Input: part model. Units: mm. Frame: model coordinates. Round coordinates to 2 decimals unless told otherwise and drop trailing zeros. Loops run counter-clockwise (first coordinate to the right, second up) from the corner with the lowest first, then second, coordinate; pieces in that order, holes last.
(1) Cut plane A-A, the plane z = -3. Output: boundary loops of the cut face in (x, y).
(2) Draft query along X for faces 1 (the face through (0.08, -17.996, -3.471)), 2 (the face through (0, -19, 1.962)), 3 (the face through (0.124, -19.995, -3.471)). Return one class per face: released by +X, released by -X, zero draft, split by the parting line, or undercut.
(3) Line query: line 1 (X direction, y = -7.5, z = -0.25); line 2 (X direction, y = -16, z = -8.25); line 3 (Y direction, x = 13.5, z = -0.5). Output: solid intervals per line, ascending.
(4) First-contact query: pin 1 Ø5 at (x, y) = (9.5, -12.5) entering from +Z; pin 2 Ø1.5 at (y, z) = (-5, -7.5) entering from -X; pin 3 Ø6 at (y, z) = (-12, -3.5) entering from -X. Flat tips, straight axial feed; report the tip coordinate or a pass-through.
from build123d import *

# Parameters (mm, degrees)
F0_W     = 2
F0_H     = 11
F2_W     = 98.8686215132
F2_H     = 62.5401474535
F3_DEPTH = 20.001
F4_R     = 0.7


with BuildPart() as f1:
    # F0 (on Front) → F1 (revolve)
    with BuildSketch(Plane.XZ):
        with Locations((18.6841351639, -3.538246952)):
            Rectangle(F0_W, F0_H)
    revolve(axis=Axis((-0.3158648361, 0, -1.3117180206), (0, 0, -1)))

    # F2 (on Front) → F3 (cut, through all)
    with BuildSketch(Plane.XZ):
        with Locations((-19.5460626855, -2.5687646121)):
            Rectangle(F2_W, F2_H)
    extrude(amount=-F3_DEPTH, mode=Mode.SUBTRACT)

    # F4
    f4_edges = [f1.edges().sort_by_distance(p)[0] for p in [
        (-0.315865, -20, 1.961753),
        (-0.315865, -18, 1.961753),
        (-0.315865, -20, -9.038247),
        (-0.315865, -18, -9.038247),
    ]]
    fillet(f4_edges, radius=F4_R)


solid = f1.part
Reported:
1. outline: (-20.32, 0) arc R20 ccw to (19.68, 0) - (17.68, 0) arc R18 cw to (-18.32, 0) - close
2. face 1: undercut
2. face 2: zero draft
2. face 3: split by the parting line
3. line 1: x = -18.86 to -16.68, 16.05 to 18.22
3. line 2: x = -12.32 to -8.56, 7.93 to 11.68
3. line 3: y = -14.46 to -11.54
4. pin 1: stops at z = 1.89
4. pin 2: stops at x = -19.86
4. pin 3: stops at x = -18.18
